For this review, use the dimensioned drawing (mm, ordinates from the lowest corner) and the shaded views. Round coordinates to 2 decimals unless told otherwise and drop trailing zeros. Order: outer loops, then holes, each group sorted by start corner. A loop starts at its lowest first (then second) coordinate and runs counter-clockwise, first axis right, second up. Notation, with made-up numbers: (-24.75, -33) -> (-5.75, -33) arc R16 cw to (-5.75, -16) -> close; hole circle Ø3 at (64.5, -36.75). An arc over 180 degrees is marked (long way). Answer in a Markdown table with one row per item.
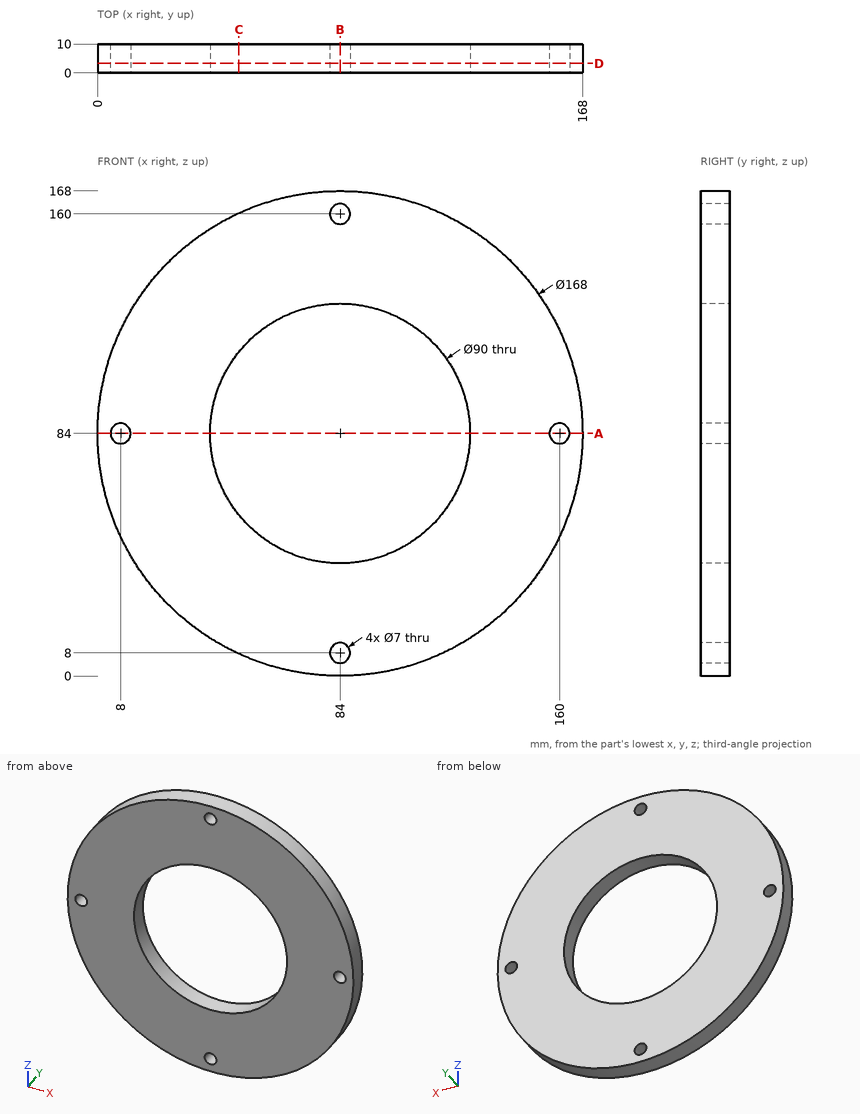
Q1. Take a section at D-D, the plane y = 3.25. Write out the cut boundary in (x, z), then the cut area to 3 significant figures.
Answer key:
| item | result |
|---|---|
| outline | circle Ø168 at (84, 84); hole circle Ø7 at (8, 84); hole circle Ø90 at (84, 84); hole circle Ø7 at (84, 8); hole circle Ø7 at (84, 160); hole circle Ø7 at (160, 84) |
| area | 15,700 mm^2 |
Q2. To check wall thickness, follow probe 1 along X at (y, z) = (7.5, 84); probe 2 along X at (y, z) = (1, 85.5) (3 decimals); probe 3 along X at (y, z) = (5.5, 93.5). State the ranges of each line that lie inside material, in increasing order.
Answer key:
| item | result |
|---|---|
| probe 1 | x = 0 to 4.5, 11.5 to 39, 129 to 156.5, 163.5 to 168 |
| probe 2 | x = 0.013 to 4.838, 11.162 to 39.025, 128.975 to 156.838, 163.162 to 167.987 |
| probe 3 | x = 0.54 to 40.01, 127.99 to 167.46 |
Q3. Take a section at B-B, the plane x = 84. Write out the cut boundary in (y, z), then the cut area to 3 significant figures.
Answer key:
| item | result |
|---|---|
| outline | (0, 0) -> (10, 0) -> (10, 4.5) -> (0, 4.5) -> close; (0, 11.5) -> (10, 11.5) -> (10, 39) -> (0, 39) -> close; (0, 129) -> (10, 129) -> (10, 156.5) -> (0, 156.5) -> close; (0, 163.5) -> (10, 163.5) -> (10, 168) -> (0, 168) -> close |
| area | 640 mm^2 |
Q4. Take a section at A-A, the plane z = 84. Write out the cut boundary in (x, y), then the cut area to 3 significant figures.
Answer key:
| item | result |
|---|---|
| outline | (0, 0) -> (4.5, 0) -> (4.5, 10) -> (0, 10) -> close; (11.5, 0) -> (39, 0) -> (39, 10) -> (11.5, 10) -> close; (129, 0) -> (156.5, 0) -> (156.5, 10) -> (129, 10) -> close; (163.5, 0) -> (168, 0) -> (168, 10) -> (163.5, 10) -> close |
| area | 640 mm^2 |
Q5. Take a section at C-C, the plane x = 49. Write out the cut boundary in (y, z).
Answer key:
| item | result |
|---|---|
| outline | (0, 7.64) -> (10, 7.64) -> (10, 55.72) -> (0, 55.72) -> close; (0, 112.28) -> (10, 112.28) -> (10, 160.36) -> (0, 160.36) -> close |
Q6. Clearance check with flat-ended pins moving along their axes: pin 1 Ø3 at (y, z) = (6, 40.5) entering from +X; pin 2 Ø5 at (x, y) = (57, 2.5) entering from -Z; pin 3 Ø6 at (x, y) = (45, 5) entering from -Z. State where each tip first meets the part, or that it passes through.
Answer key:
| item | result |
|---|---|
| pin 1 | stops at x = 156.75 |
| pin 2 | stops at z = 3.65 |
| pin 3 | stops at z = 8.11 |
